Geometry check sheet. Reference: the model listing, model coordinates, mm. Face numbers are marked on the shaded views. A direction names the side the tool comes from. Round coordinates to 2 decimals unless told otherwise and drop trailing zeros. Order: outer loops, then holes, each group sorted by start corner. A loop starts at its lowest first (then second) coordinate and runs counter-clockwise, first axis right, second up. Notation, with made-up numbers: (77.5, 8) -> (135.5, 8) arc R29 ccw to (135.5, 31) -> close; hole circle Ø3 at (-9, -4.75). An arc over 180 degrees is marked (long way). Use a Markdown table: item, result. Add a question column.
Item 1: Sectioned sample at A-A, the plane x = 0. Record the cut outline in (y, z).
Item 2: Sectioned sample at B-B, the plane z = 1.5. Record the cut outline in (x, y).
Item 3: Material ranges on probe 1 along X at (y, z) = (1.2, 0); probe 2 along Y at (x, z) = (1.5, -4); probe 3 along Z at (x, y) = (-3.5, 17), recorded low to high. Write a range as [from, to].
Item 4: Sectioned sample at C-C, the plane x = -6. Record the cut outline in (y, z).
Item 5: Set-up check for the marked faces 1 and 2: record each of +Z, -Z, +X, -X, +Y, -Y from which the full face is reachable in a straight line by a thin tool's end or side.
Item 6: Sectioned sample at D-D, the plane z = -9. Record the cut outline in (x, y), and give its area (3 significant figures).
Item 7: Gauge pin test, flat ends, axial feed: pin 1 Ø3 at (x, y) = (-4.5, 28) entering from -Z; pin 2 Ø10 at (x, z) = (6.5, -8) entering from +Y; pin 3 Ø3 at (x, z) = (0, 0) entering from -Y; pin 4 Ø4 at (x, y) = (-3, 11.5) entering from -Z. Record the tip position at first contact, or that the pin passes through.
from build123d import *

# Parameters (mm, degrees)
SKETCH1_R           = 2.5
BOSS_EXTRUDE1_DEPTH = 2
BOSS_EXTRUDE3_DEPTH = 21


with BuildPart() as part:
    # Sketch1 → Boss-Extrude1 (new body)
    with BuildSketch(Plane(origin=(0, 0, 0), x_dir=(1, 0, 0), z_dir=(0, 1, 0))):
        with BuildLine():
            Line((-10.5, 0), (-10.5, 10))
            Line((-10.5, 10), (10.5, 10))
            Line((10.5, 10), (10.5, 0))
            ThreePointArc((10.5, 0), (0, -10.5), (-10.5, 0))
        make_face()
        with Locations(Location((0, 0, 0), (0, 0, 270))):
            Circle(SKETCH1_R, mode=Mode.SUBTRACT)
    extrude(amount=BOSS_EXTRUDE1_DEPTH)

    # Sketch3 → Boss-Extrude3 (add)
    with BuildSketch(Plane(origin=(10.5, 0, 0), x_dir=(0, 0, -1), z_dir=(1, 0, 0))):
        Polygon((10, 0), (19.91, 19.2), (28.065104167, 35), (25.39926045, 36.375964127), (6.623958132, 0), align=None)
    extrude(amount=-BOSS_EXTRUDE3_DEPTH)


solid = part.part
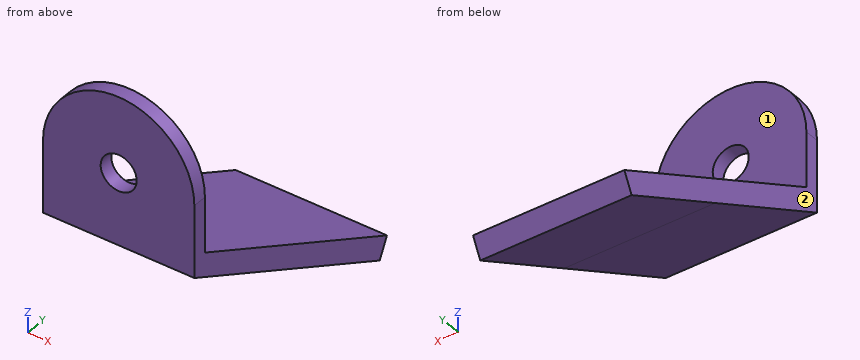
Found:
| question | item | result |
|---|---|---|
| 1 | outline | (0, -10) -> (35, -28.07) -> (36.38, -25.4) -> (2, -7.66) -> (2, -2.5) -> (0, -2.5) -> close; (0, 2.5) -> (2, 2.5) -> (2, 10.5) -> (0, 10.5) -> close |
| 2 | outline | (-10.39, 0) -> (-2, 0) -> (-2, 2) -> (-10.39, 2) -> close; (2, 0) -> (10.39, 0) -> (10.39, 2) -> (2, 2) -> close |
| 3 | probe 1 | x = [-10.5, -2.5], [2.5, 10.5] |
| 3 | probe 2 | y = [0, 2] |
| 3 | probe 3 | z = [-18.77, -15.4] |
| 4 | outline | (0, -10) -> (35, -28.07) -> (36.38, -25.4) -> (2, -7.66) -> (2, 8.62) -> (0, 8.62) -> close |
| 5 | face 1 | +Z, +X, -X, +Y |
| 5 | face 2 | +Z, -Z, -X, +Y, -Y |
| 6 | outline | (-10.5, 0) -> (10.5, 0) -> (10.5, 4.6) -> (-10.5, 4.6) -> close |
| 6 | area | 96.7 mm2 |
| 7 | pin 1 | stops at z = -25.23 |
| 7 | pin 2 | stops at y = 12.35 |
| 7 | pin 3 | passes through |
| 7 | pin 4 | stops at z = -16.97 |
